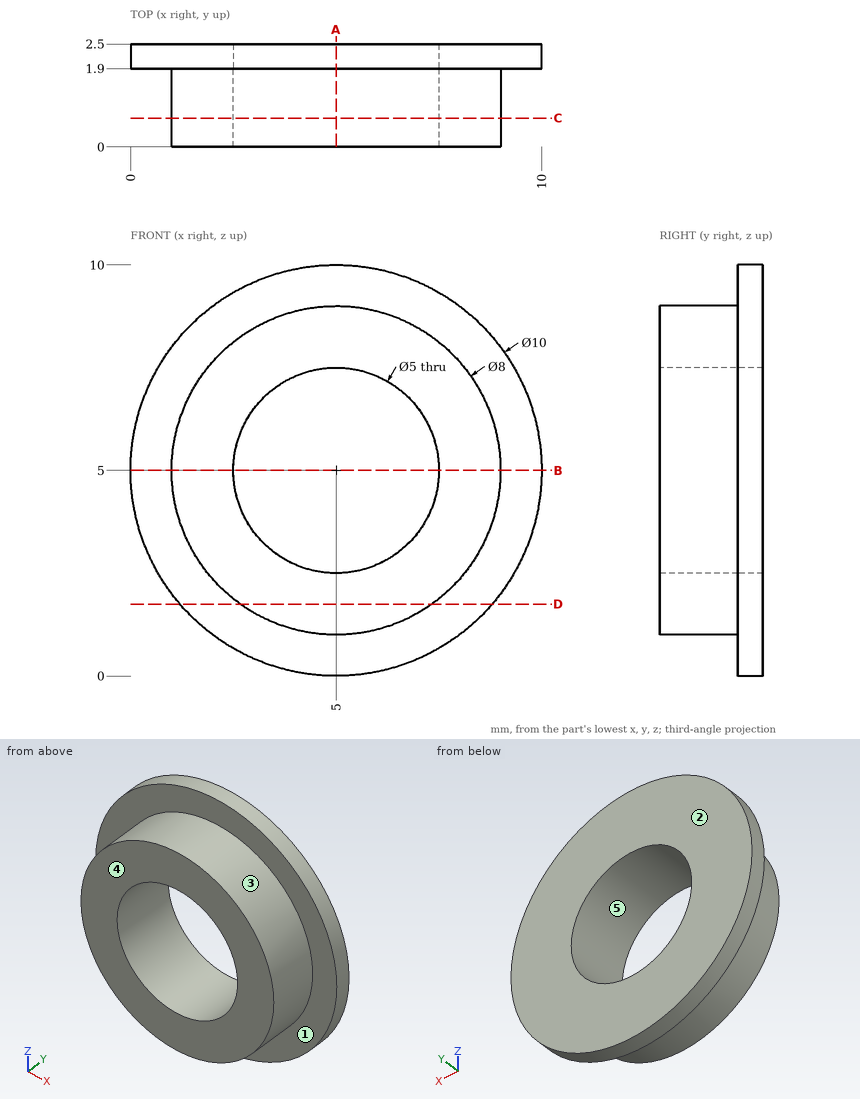
Job drawing, mm, ordinate dimensions from the low corner. One solid piece. A direction names the side the tool comes from. Give positions to 0.01 mm unless a question says otherwise; leave off trailing zeros. Loops run counter-clockwise (first coordinate to the right, second up) from the corner with the lowest first, then second, coordinate; pieces in that order, holes last. Notation, with made-up numbers: (-6, 61) -> (43, 61) arc R21 ccw to (43, 67) -> close; hole circle Ø2 at (89.25, 11.25). An arc over 180 degrees is marked (long way). Write each question's results on one line, items separated by ' | '. Start each with the question number.
Q1. Which spindle directions (+Z, -Z, +X, -X, +Y, -Y) get a long thin tool onto all of the face, cutting with end or side? Do the marked faces 1 and 2. Say none if no direction does.
Q2. Band-saw the part on B-B on z = 5. List the corners of the cut face in (x, y), plus the area to 3 significant figures.
Q3. Band-saw the part on A-A on x = 5. List the corners of the cut face in (y, z).
Q4. Band-saw the part on C-C on y = 0.7. List the corners of the cut face in (x, z).
Q5. Pull direction Z, two halves, no side cores. Call the marked faces 3, 4 and 5: +Z half, -Z half, draft (parallel to the pull), parting line (faces both ways), or undercut.
Q6. Pin check, flat tip, straight feed: P1, Ø1, axis at x = 2.5, y = 2, coming from the +Z side. Stop position of the tip, or through.
Q7. Wall check: L1, parallel to X at y = 2.05, z = 5; L2, parallel to Z at x = 5, y = 1. Give the ranges that are in metal, low to high.
Q8. Band-saw the part on D-D on z = 1.75. List the corners of the cut face in (x, y).
Results are:
1) face 1: -Y | face 2: +Z, -Z, +X, -X, +Y
2) outline: (0, 1.9) -> (1, 1.9) -> (1, 0) -> (2.5, 0) -> (2.5, 2.5) -> (0, 2.5) -> close; (7.5, 0) -> (9, 0) -> (9, 1.9) -> (10, 1.9) -> (10, 2.5) -> (7.5, 2.5) -> close | area: 8.70 mm²
3) outline: (0, 1) -> (1.9, 1) -> (1.9, 0) -> (2.5, 0) -> (2.5, 2.5) -> (0, 2.5) -> close; (0, 7.5) -> (2.5, 7.5) -> (2.5, 10) -> (1.9, 10) -> (1.9, 9) -> (0, 9) -> close
4) outline: circle Ø8 at (5, 5); hole circle Ø5 at (5, 5)
5) face 3: parting line | face 4: draft | face 5: undercut
6) P1: stops at z = 9.58
7) L1: x = 0 to 2.5, 7.5 to 10 | L2: z = 1 to 2.5, 7.5 to 9
8) outline: (1.2, 1.9) -> (2.67, 1.9) -> (2.67, 0) -> (7.33, 0) -> (7.33, 1.9) -> (8.8, 1.9) -> (8.8, 2.5) -> (1.2, 2.5) -> close
